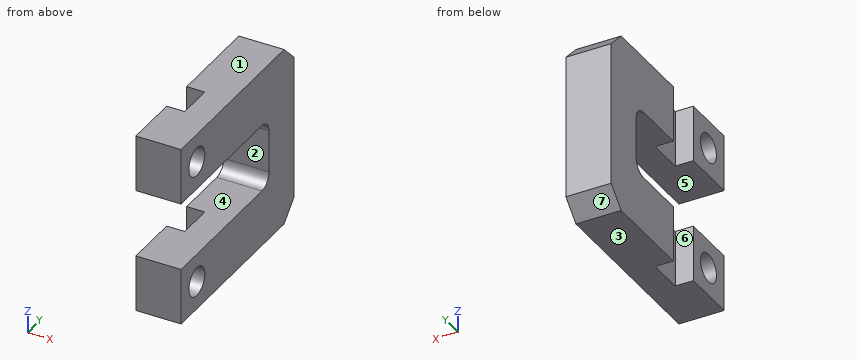
```python
from build123d import *

# Parameters (mm, degrees)
BOSS_EXTRUDE1_DEPTH    = 6.35
F_10_32_TAPPED_HOLE1_D = 4.0386
SKETCH2_W              = 25.4
SKETCH2_H              = 5.08
CUT_EXTRUDE1_DEPTH     = 2.54
CHAMFER1_SIZE          = 2.54


with BuildPart() as part:
    # Sketch1 → Boss-Extrude1 (new body)
    with BuildSketch(Plane(origin=(0, 0, 0), x_dir=(0, 0, -1), z_dir=(1, 0, 0))):
        with BuildLine():
            Line((7.9375, 0), (7.9375, 20.447))
            ThreePointArc((7.9375, 20.447), (8.458264143, 21.704235857), (9.7155, 22.225))
            Line((9.7155, 22.225), (15.6845, 22.225))
            ThreePointArc((15.6845, 22.225), (16.941735857, 21.704235857), (17.4625, 20.447))
            Line((17.4625, 20.447), (17.4625, 0))
            Line((17.4625, 0), (25.4, 0))
            Line((25.4, 0), (25.4, 28.575))
            Line((25.4, 28.575), (0, 28.575))
            Line((0, 28.575), (0, 0))
            Line((0, 0), (7.9375, 0))
        make_face()
    extrude(amount=BOSS_EXTRUDE1_DEPTH)

    # #10-32 Tapped Hole1 (through all)
    with Locations(Plane.ZY):
        with Locations((-21.43125, 3.96875), (-3.96875, 3.96875)):
            Hole(F_10_32_TAPPED_HOLE1_D / 2)

    # Sketch2 → Cut-Extrude1 (cut)
    with BuildSketch(Plane.ZY):
        with Locations((-12.7, 10.31875)):
            Rectangle(SKETCH2_W, SKETCH2_H)
    extrude(amount=-CUT_EXTRUDE1_DEPTH, mode=Mode.SUBTRACT)

    # Chamfer1
    chamfer1_edges = [part.edges().sort_by_distance(p)[0] for p in [
        (3.175, 28.575, 0),
        (3.175, 28.575, -25.4),
    ]]
    chamfer(chamfer1_edges, length=CHAMFER1_SIZE)


solid = part.part
```
Geometry: final body of the model. Coordinates: model frame, mm. Face numbers are marked on the shaded views. A direction names the side the tool comes from. Give positions to 0.01 mm unless a question says otherwise; leave off trailing zeros. Order: outer loops, then holes, each group sorted by start corner. A loop starts at its lowest first (then second) coordinate and runs counter-clockwise, first axis right, second up. Notation, with made-up numbers: M 27,-1.5 L 61,-1.5 A32 cw 61,30.5 Z; hole C 17.5,76.5 d5. An arc over 180 degrees is marked long. Answer as CSV lines item,"result". Start each with the question number.
1) Line query: line 1 (Y direction, x = 0.75, z = -21.5) (3 decimals); line 2 (Z direction, x = 4.5, y = 7); line 3 (Y direction, x = 2.75, z = -12.5) (3 decimals). Output: solid intervals per line, ascending. Write a range as from..to.
2) Cut plane B-B (y = 14). Output: boundary loops of the cut face in (x, z).
3) Cut plane C-C (z = -22). Output: boundary loops of the cut face in (x, y) (3 decimals).
4) Set-up query: the marked faces 5, 6 and 7. Return all of +Z, -Z, +X, -X, +Y, -Y with unobstructed straight access to the full face (end or side cutting, diameter ignored); none if empty.
5) Cut plane D-D (y = 3). Output: boundary loops of the cut face in (x, z), then the cut area to 3 significant figures.
6) Mould query, pull axis Z, two halves, no side actions, for the marked faces 1, 2, 3 and 4. Classes: +Z half, -Z half, draft (parallel to the pull), parting line (faces both ways), or undercut.
7) Cut plane A-A (x = 1.75). Output: boundary loops of the cut face in (y, z) (1 decimal).
8) First-contact query: P1, Ø3, axis at x = 1.5, z = -12, coming from the -Y side (3 decimals); P2, Ø2.5, axis at y = 10, z = -20.5, coming from the -X side. Flat tips, straight axial feed; report the tip coordinate or a pass-through.
Findings below:
1,line 1,"y = 0..1.951, 5.987..7.779, 12.859..28.575"
1,line 2,"z = -25.4..-17.46, -7.94..0"
1,line 3,"y = 22.225..28.575"
2,outline,"M 0,-25.4 L 6.35,-25.4 L 6.35,-17.46 L 0,-17.46 Z; M 0,-7.94 L 6.35,-7.94 L 6.35,0 L 0,0 Z"
3,outline,"M 0,0 L 6.35,0 L 6.35,2.031 L 0,2.031 Z; M 0,5.906 L 6.35,5.906 L 6.35,28.575 L 0,28.575 L 0,12.859 L 2.54,12.859 L 2.54,7.779 L 0,7.779 Z"
4,face 5,"+X, -X, -Y"
4,face 6,"+Z, -Z, -X"
4,face 7,"-Z, +X, -X, +Y"
5,outline,"M 0,-25.4 L 6.35,-25.4 L 6.35,-23.2 L 0,-23.2 Z; M 0,-19.66 L 6.35,-19.66 L 6.35,-17.46 L 0,-17.46 Z; M 0,-7.94 L 6.35,-7.94 L 6.35,-5.74 L 0,-5.74 Z; M 0,-2.2 L 6.35,-2.2 L 6.35,0 L 0,0 Z"
5,area,"55.8 mm²"
6,face 1,"+Z half"
6,face 2,"undercut"
6,face 3,"-Z half"
6,face 4,"undercut"
7,outline,"M 0,-25.4 L 7.8,-25.4 L 7.8,-17.5 L 0,-17.5 Z; M 0,-7.9 L 7.8,-7.9 L 7.8,0 L 0,0 Z; M 12.9,-25.4 L 26,-25.4 L 28.6,-22.9 L 28.6,-2.5 L 26,0 L 12.9,0 L 12.9,-7.9 L 20.4,-7.9 A1.8 cw 22.2,-9.7 L 22.2,-15.7 A1.8 cw 20.4,-17.5 L 12.9,-17.5 Z; hole C 4,-21.4 d4; hole C 4,-4 d4"
8,P1,"stops at y = 22.225"
8,P2,"stops at x = 2.54"
